Geometry check sheet. Reference: drawing and pictorial views, mm from the part's lowest x, y, z. Give positions to 0.01 mm unless a question says otherwise; leave off trailing zeros. Order: outer loops, then holes, each group sorted by start corner. A loop starts at its lowest first (then second) coordinate and runs counter-clockwise, first axis right, second up.
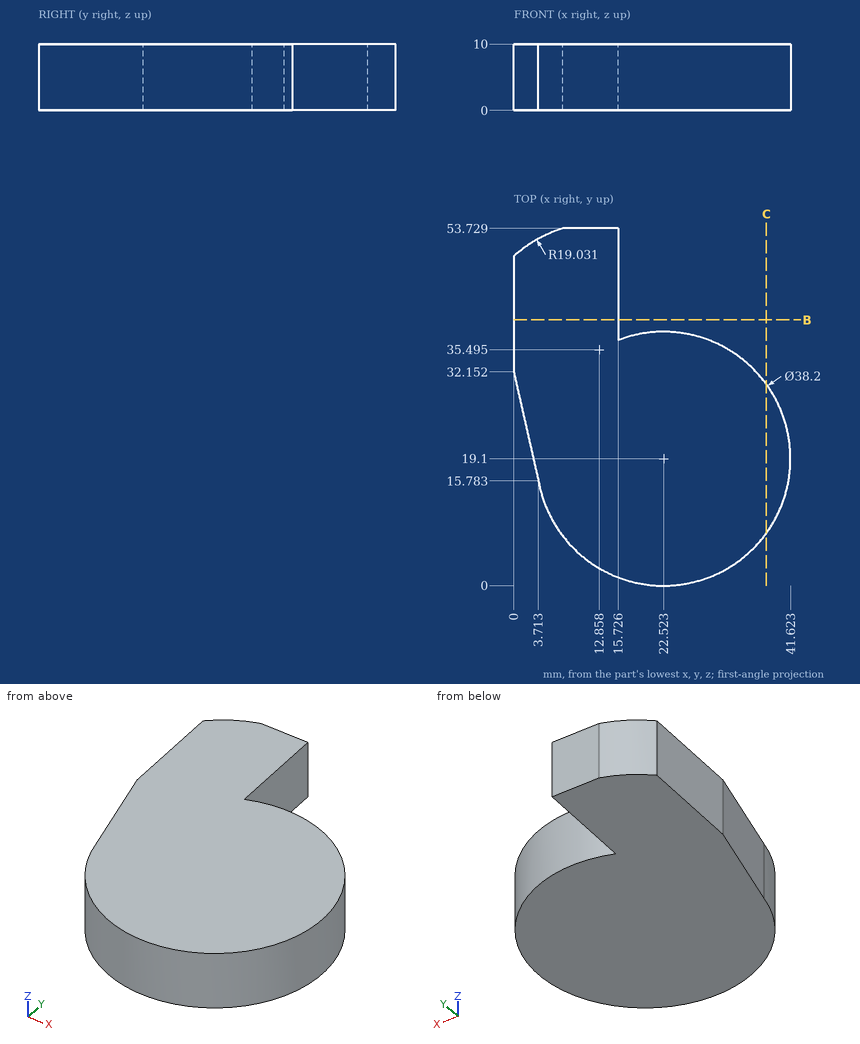
1) Depth check by flat-ended pin: pin 1 Ø3 at (y, z) = (45, 2) entering from +X; pin 2 Ø10 at (x, y) = (30.5, 43.5) entering from +Z. Enter the tip coordinate at first touch or a pass-through.
Recorded:
pin 1: stops at x = 15.73
pin 2: passes through
2) Section check C-C, the plane x = 38. Record the cut outline in (y, z).
Recorded:
outline: (7.91, 0) - (30.29, 0) - (30.29, 10) - (7.91, 10) - close
3) Section check B-B, the plane y = 40. Record the cut outline in (x, z), then the cut area to 3 significant figures.
Recorded:
outline: (0, 0) - (15.73, 0) - (15.73, 10) - (0, 10) - close
area: 157 mm2
4) Material ranges on L1, parallel to X at y = 48, z = 3.75; L2, parallel to Y at x = 22.5, z = 2.75; L3, parallel to X at y = 11.5, z = 1.5 (1 decimal), recorded low to high.
Recorded:
L1: x = 0 to 15.73
L2: y = 0 to 38.2
L3: x = 5 to 40
